from build123d import *

# Parameters (mm, degrees)
SKETCH_2_W          = 11.803502198
SKETCH_2_H          = 1.437820381
CUT_EXTRUDE_1_DEPTH = 10


with BuildPart() as part:
    # Эскиз1 → Повернуть1 (revolve)
    with BuildSketch(Plane.XY, mode=Mode.PRIVATE) as revolve_1_sk:
        Polygon((-1.25, 0), (-2.25, 0), (-2.25, 7), (-6, 7), (-6, 9), (-2, 9), (-2, 14), (-2.75, 14), (-2, 19), (-1.25, 19), align=None)
    revolve(revolve_1_sk.sketch.rotate(Axis((0, 0, 0), (0, 1, 0)), 270), axis=Axis((0, 0, 0), (0, 1, 0)))

    # Эскиз2 → Вырез-Вытянуть1 (cut)
    with BuildSketch(Plane(origin=(0, 9, 0), x_dir=(1, 0, 0), z_dir=(0, 1, 0))):
        with Locations((0, -5.718910191)):
            Rectangle(SKETCH_2_W, SKETCH_2_H)
        with Locations((0, 5.718910191)):
            Rectangle(SKETCH_2_W, SKETCH_2_H)
    extrude(amount=-CUT_EXTRUDE_1_DEPTH, mode=Mode.SUBTRACT)


solid = part.part
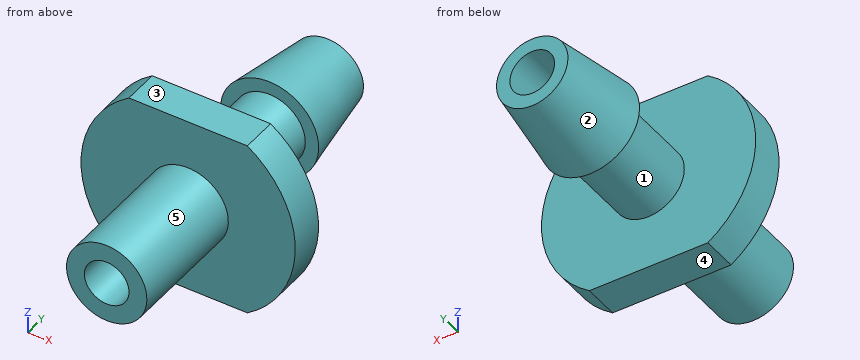
Could you check a few things on this model? Use its own coordinates, in mm. Face numbers are marked on the shaded views. A direction names the side the tool comes from. Give positions to 0.01 mm unless a question says otherwise; leave off trailing zeros. Order: outer loops, then holes, each group sorted by start corner. A loop starts at its lowest first (then second) coordinate and runs counter-clockwise, first axis right, second up. Notation, with made-up numbers: (-25, -14.75) - (30, -14.75) arc R28 ccw to (30, 23.25) - close; hole circle Ø10 at (17.5, -17.5). An arc over 180 degrees is marked (long way). One line per item, written item: value. Start each with the question number.
1. Thinking about a two-plate mould opening in Y: for the marked faces 1, 2 and 3, which applies, +Y half, -Y half, draft (parallel to the pull), parting line (faces both ways), or undercut?
2. For the marked faces 4 and 5, which set-ups out of +Z, -Z, +X, -X, +Y, -Y let a thin tool reach every point of the face, with its end or its side?
3. If I drill on probe 1 along X at (y, z) = (8.75, 0); probe 2 along X at (y, z) = (11, 0); probe 3 along Y at (x, z) = (0, 3.25), over which ranges is the centre line in solid material (lowest first)?
4. Imagine slicing it at D-D on y = 3. List the corners of the cut face in (x, z) for me.
5. Imagine slicing it at A-A on z = 0. List the corners of the cut face in (x, y) for me.
6. For P1, Ø1, axis at x = -1, z = -3, coming from the -Y side; P2, Ø5, axis at y = 12, z = -3.5, coming from the +X side; P3, Ø3, axis at y = 17, z = 3, coming from the +X side, each with a flat end and sliding along its axis, tell me the tip position at first contact or that it passes through.
7. Imagine slicing it at C-C on x = 0. List the corners of the cut face in (y, z) for me, plus the area to 4 significant figures.
8. Imagine slicing it at B-B on y = 8.25. List the corners of the cut face in (x, z) for me, plus the area to 3 significant figures.
Values:
1. face 1: undercut
1. face 2: +Y half
1. face 3: draft
2. face 4: -Z, +X, -X, +Y, -Y
2. face 5: -Y
3. probe 1: -6 to -1.25, 1.25 to 6
3. probe 2: -2 to -1.25, 1.25 to 2
3. probe 3: 7 to 9
4. outline: circle Ø4.5 at (0, 0); hole circle Ø2.5 at (0, 0)
5. outline: (-6, 7) - (-2.25, 7) - (-2.25, 0) - (-1.25, 0) - (-1.25, 19) - (-2, 19) - (-2.75, 14) - (-2, 14) - (-2, 9) - (-6, 9) - close; (1.25, 0) - (2.25, 0) - (2.25, 7) - (6, 7) - (6, 9) - (2, 9) - (2, 14) - (2.75, 14) - (2, 19) - (1.25, 19) - close
6. P1: y = 7
6. P2: x = 1.89
6. P3: x = 1.78
7. outline: (0, -2.25) - (7, -2.25) - (7, -5) - (9, -5) - (9, -2) - (14, -2) - (14, -2.75) - (19, -2) - (19, -1.25) - (0, -1.25) - close; (0, 1.25) - (19, 1.25) - (19, 2) - (14, 2.75) - (14, 2) - (9, 2) - (9, 5) - (7, 5) - (7, 2.25) - (0, 2.25) - close
7. area: 47.75 mm²
8. outline: (-3.32, -5) - (3.32, -5) arc R6 ccw to (3.32, 5) - (-3.32, 5) arc R6 ccw to start; hole circle Ø2.5 at (0, 0)
8. area: 99.2 mm²
